For this review, take the finished solid that the model builds, in its own axes (mm). Coordinates: 2 decimals unless noted, no trailing zeros. Loops run counter-clockwise (first coordinate to the right, second up) from the corner with the lowest first, then second, coordinate; pieces in that order, holes last. Notation, with made-up numbers: (36.25, 36.25) - (87.25, 36.25) arc R27 cw to (87.25, 63.25) - close; hole circle Ø4 at (45, -0.75). An arc over 180 degrees is marked (long way). One line per item, written item: value. Start each with the question number.
1. Take a section at C-C, the plane z = 20.8. State the section outline as (x, y) points, and give its area (3 significant figures).
2. To check wall thickness, follow line 1 (X direction, y = 2, z = -20.8); line 2 (X direction, y = 4.75, z = 20.8); line 3 (Y direction, x = 21, z = -16). State the ranges of each line that lie inside material, in increasing order. Write a range as from..to.
3. Take a section at D-D, the plane z = -24.5. State the section outline as (x, y) points.
4. Insertion check: pin 1 (4.5 mm diameter, centred on x = -39, z = -24.5, fed in from +Y); pin 2 (4.5 mm diameter, centred on x = 0, z = 20.8, fed in from +Y); pin 3 (4 mm diameter, centred on y = 8.5, z = -3, fed in from -X); pin 4 (1.2 mm diameter, centred on x = -18.5, z = 0.5, fed in from +Y). Each pin has a flat end and moves straight along its axis. Give the tip position at first contact, or say it passes through.
5. Take a section at B-B, the plane x = 19. State the section outline as (y, z) points, and give its area (3 significant figures).
6. Take a section at A-A, the plane y = 5.25. State the section outline as (x, z) points.
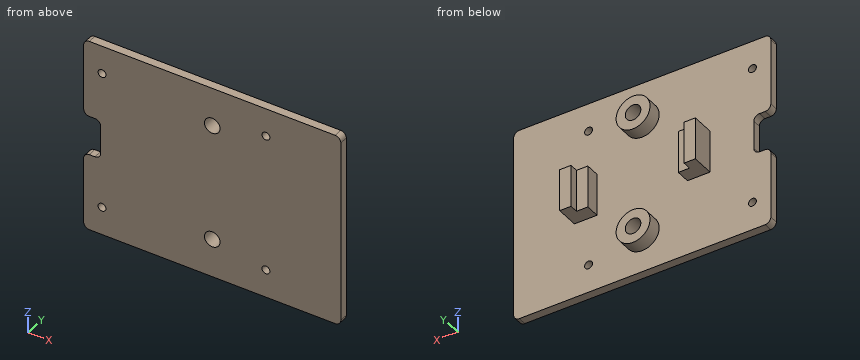
```python
from build123d import *

# Parameters (mm, degrees)
SKETCH1_W           = 91
SKETCH1_H           = 69
BOSS_EXTRUDE1_DEPTH = 3
SKETCH2_W           = 6
SKETCH2_H           = 14
CUT_EXTRUDE1_DEPTH  = 58.179541796
SKETCH3_R           = 1.4
CUT_EXTRUDE2_DEPTH  = 58.179541796
FILLET1_R           = 2
SKETCH6_R           = 6
SKETCH6_W           = 8
SKETCH6_H           = 15
BOSS_EXTRUDE2_DEPTH = 5
SKETCH5_R           = 2.75
CUT_EXTRUDE3_DEPTH  = 58.658477261
SKETCH7_W           = 4
SKETCH7_H           = 15
BOSS_EXTRUDE3_DEPTH = 3


with BuildPart() as part:
    # Sketch1 → Boss-Extrude1 (new body)
    with BuildSketch(Plane(origin=(0, 0, 0), x_dir=(1, 0, 0), z_dir=(0, 1, 0))):
        Rectangle(SKETCH1_W, SKETCH1_H)
    extrude(amount=BOSS_EXTRUDE1_DEPTH)

    # Sketch2 → Cut-Extrude1 (cut, through all)
    with BuildSketch(Plane(origin=(0, 3, 0), x_dir=(1, 0, 0), z_dir=(0, 1, 0))):
        with Locations((-42.5, 0)):
            Rectangle(SKETCH2_W, SKETCH2_H)
    extrude(amount=-CUT_EXTRUDE1_DEPTH, mode=Mode.SUBTRACT)

    # Sketch3 → Cut-Extrude2 (cut, through all)
    with BuildSketch(Plane(origin=(0, 3, 0), x_dir=(1, 0, 0), z_dir=(0, 1, 0))):
        with Locations(Location((-39, 24.5, 0), (0, 0, 270))):
            Circle(SKETCH3_R)
        with Locations(Location((19, 24.5, 0), (0, 0, 270))):
            Circle(SKETCH3_R)
        with Locations(Location((19, -24.5, 0), (0, 0, 90))):
            Circle(SKETCH3_R)
        with Locations(Location((-39, -24.5, 0), (0, 0, 90))):
            Circle(SKETCH3_R)
    extrude(amount=-CUT_EXTRUDE2_DEPTH, mode=Mode.SUBTRACT)

    # Fillet1
    fillet1_edges = [part.edges().sort_by_distance(p)[0] for p in [
        (-45.5, 1.5, 7),
        (-45.5, 1.5, -7),
        (-39.5, 1.5, -7),
        (-39.5, 1.5, 7),
        (45.5, 1.5, 34.5),
        (-45.5, 1.5, 34.5),
        (-45.5, 1.5, -34.5),
        (45.5, 1.5, -34.5),
    ]]
    fillet(fillet1_edges, radius=FILLET1_R)

    # Sketch6 → Boss-Extrude2 (add)
    with BuildSketch(Plane(origin=(0, 3, 0), x_dir=(1, 0, 0), z_dir=(0, 1, 0))):
        with Locations(Location((0, -20.8, 0), (0, 0, 270))):
            Circle(SKETCH6_R)
        with Locations(Location((0, 20.8, 0), (0, 0, 270))):
            Circle(SKETCH6_R)
        with Locations((-20, 0)):
            Rectangle(SKETCH6_W, SKETCH6_H)
        with Locations((20, 0)):
            Rectangle(SKETCH6_W, SKETCH6_H)
    extrude(amount=BOSS_EXTRUDE2_DEPTH)

    # Sketch5 → Cut-Extrude3 (cut, through all)
    with BuildSketch(Plane(origin=(0, 0, 0), x_dir=(-1, 0, 0), z_dir=(0, -1, 0))):
        with Locations(Location((0, -20.8, 0), (0, 0, 90))):
            Circle(SKETCH5_R)
        with Locations(Location((0, 20.8, 0), (0, 0, 90))):
            Circle(SKETCH5_R)
    extrude(amount=-CUT_EXTRUDE3_DEPTH, mode=Mode.SUBTRACT)

    # Sketch7 → Boss-Extrude3 (add)
    with BuildSketch(Plane(origin=(0, 8, 0), x_dir=(1, 0, 0), z_dir=(0, 1, 0))):
        with Locations((22, 0)):
            Rectangle(SKETCH7_W, SKETCH7_H)
        with Locations((-22, 0)):
            Rectangle(SKETCH7_W, SKETCH7_H)
    extrude(amount=BOSS_EXTRUDE3_DEPTH)


solid = part.part
```
Solutions:
1. outline: (-45.5, 0) - (-2.75, 0) - (-2.75, 8) - (-6, 8) - (-6, 3) - (-45.5, 3) - close; (2.75, 0) - (45.5, 0) - (45.5, 3) - (6, 3) - (6, 8) - (2.75, 8) - close
1. area: 289 mm2
2. line 1: -45.5..-2.75, 2.75..45.5
2. line 2: -6..-2.75, 2.75..6
2. line 3: 0..3
3. outline: (-45.5, 0) - (-40.4, 0) - (-40.4, 3) - (-45.5, 3) - close; (-37.6, 0) - (17.6, 0) - (17.6, 3) - (4.72, 3) - (4.72, 8) - (-4.72, 8) - (-4.72, 3) - (-37.6, 3) - close; (20.4, 0) - (45.5, 0) - (45.5, 3) - (20.4, 3) - close
4. pin 1: y = 3
4. pin 2: through
4. pin 3: x = -24
4. pin 4: y = 8
5. outline: (0, -34.5) - (3, -34.5) - (3, -25.9) - (0, -25.9) - close; (0, -23.1) - (3, -23.1) - (3, -7.5) - (8, -7.5) - (8, 7.5) - (3, 7.5) - (3, 23.1) - (0, 23.1) - close; (0, 25.9) - (3, 25.9) - (3, 34.5) - (0, 34.5) - close
5. area: 265 mm2
6. outline: (-24, -7.5) - (-16, -7.5) - (-16, 7.5) - (-24, 7.5) - close; circle Ø12 at (0, -20.8); circle Ø12 at (0, 20.8); (16, -7.5) - (24, -7.5) - (24, 7.5) - (16, 7.5) - close; hole circle Ø5.5 at (0, -20.8); hole circle Ø5.5 at (0, 20.8)
